Could you check a few things on this model? Use its own coordinates, in mm. A direction names the side the tool comes from. Give positions to 0.01 mm unless a question says otherwise; leave off trailing zeros. Loops run counter-clockwise (first coordinate to the right, second up) from the corner with the lowest first, then second, coordinate; pieces in that order, holes last. Notation, with made-up numbers: (52.5, 25.25) - (77.5, 25.25) arc R20 cw to (77.5, 58.25) - close; hole circle Ø5 at (58, 88). An arc over 180 degrees is marked (long way). Write each question's results on one line, items separated by ' | '. Start each with the question number.
(1) Suppose I cut it at A-A (x = -39). Please give me the cut outline in (y, z).
(2) For pin 1 (1.8 mm diameter, centred on y = 1.5, z = 12, fed in from -X); pin 2 (10 mm diameter, centred on x = -12.5, z = 27.5, fed in from -Y); pin 3 (3 mm diameter, centred on y = 4, z = 47, fed in from +X); pin 4 (1.8 mm diameter, centred on x = -40.5, y = 4.5, fed in from +Z), each with a flat end and sliding along its axis, tell me the tip position at first contact or that it passes through.
(3) Suppose I cut it at C-C (x = 10.5). Please give me the cut outline in (y, z).
(4) I need wall thicknesses on line 1 (Z direction, x = -1.5, y = 3.7); line 2 (Z direction, x = -11.7, y = 4.4); line 3 (Z direction, x = 10.5, y = 1.55). Which ranges of each line are inside material? Lowest first, please.
(5) Suppose I cut it at B-B (x = -11.7). Please give me the cut outline in (y, z).
(6) On a 3-axis mill with a long thin cutter (end or side, diameter ignored), from which of +Z, -Z, +X, -X, +Y, -Y can I reach the whole of each face in a straight line? I mean faces 4 (the face through (-33, 3, 27)), 5 (the face through (-38, 3, 13)), 6 (the face through (0, 3, 54)), 7 (the face through (0, 3, 3)), 8 (the face through (7, 3, 20)). Say none if no direction works.
(7) Suppose I cut it at D-D (z = 30.5). Please give me the cut outline in (x, y), and give its area (3 significant figures).
(8) If we mould it in two halves opening along X, with no side actions, what happens to faces 1 (the face through (19, 3, 31)), 2 (the face through (-41, 3, 21)), 3 (the face through (10.37, 3.042, 37.545))? For each: released by +X, released by -X, zero draft, split by the parting line, or undercut.
Autodesk Inventor part; units mm, degrees
ref_plane "YZ Plane" through (0, 0, 0) normal (1, 0, 0) x (0, 1, 0)
ref_plane "XZ Plane" through (0, 0, 0) normal (0, 1, 0) x (-1, 0, 0)
ref_plane "XY Plane" through (0, 0, 0) normal (0, 0, 1) x (1, 0, 0)
sketch "Sketch1" plane through (0, 0, 0) normal (0, 1, 0) x (-1, 0, 0)
  line L0 (0, 0) -> (38, 0)
  line L1 (44, 0) -> (44, 6)
  line L2 (44, 27) -> (38, 27)
  line L3 (0, 27) -> (0, 6) construction
  line L4 (44, 27) -> (38, 27)
  line L5 (38, 27) -> (38, 21) construction
  line L6 (38, 21) -> (44, 21)
  line L7 (44, 21) -> (44, 27)
  line L8 (44, 0) -> (38, 0)
  line L9 (38, 0) -> (38, 6) construction
  line L10 (38, 6) -> (44, 6)
  line L11 (44, 6) -> (44, 0)
  line L12 (44, 21) -> (44, 27)
  line L13 (38, 27) -> (6, 27)
  line L14 (38, 0) -> (44, 0)
  line L15 (44, 6) -> (44, 21) construction
  line L16 (38, 6) -> (38, 21)
  line L17 (0, 0) -> (6, 0)
  line L18 (6, 0) -> (6, 6) construction
  line L19 (6, 6) -> (0, 6)
  line L20 (0, 6) -> (0, 0)
  line L21 (6, 6) -> (6, 27)
  line L22 (6, 27) -> (0, 27) construction
  line L23 (0, 6) -> (0, 0)
  line L24 (6, 27) -> (21, 27)
  line L25 (21, 27) -> (21, 57)
  line L26 (21, 57) -> (6, 57)
  line L27 (6, 57) -> (0, 57)
  line L28 (0, 57) -> (0, 51)
  line L29 (0, 51) -> (6, 51)
  line L30 (6, 51) -> (6, 57) construction
  line L31 (6, 51) -> (6, 27)
  line L32 (6, 42) -> (-19, 42)
  line L33 (-19, 42) -> (-19, 20)
  line L34 (-19, 20) -> (6, 20)
  line L35 (6, 20) -> (6, 42)
  dimension "d0" = 44
  dimension "d1" = 27
  dimension "d2" = 6
  dimension "d3" = 6
  dimension "d4" = 6
  dimension "d5" = 6
  dimension "d6" = 6
  dimension "d7" = 6
  dimension "d10" = 15
  dimension "d11" = 30
  dimension "d12" = 6
  dimension "d13" = 6
  dimension "d34" = 25
  dimension "d35" = 22
  dimension "d36" = 9
extrude "Extrusion1" add sketch "Sketch1" along normal blind 6
sketch "Sketch2" plane through (0, 6, 0) normal (0, 1, 0) x (1, 0, 0)
  circle A0 centre (10.5, -38.536) radius 1
  circle A1 centre (10.5, -35.536) radius 1
  circle A2 centre (10.5, -32.536) radius 1
  circle A3 centre (-11.7, -28.236) radius 1
  circle A4 centre (-11.7, -25.236) radius 1
  circle A5 centre (-11.7, -22.236) radius 1
  line L0 (0, -51) -> (-6, -51)
  line L1 (19, -42) -> (19, -20)
  dimension "d22" = 2
  dimension "d24" = 2
  dimension "d25" = 3
  dimension "d26" = 2
  dimension "d27" = 3
  dimension "d28" = 2
  dimension "d29" = 2
  dimension "d30" = 3
  dimension "d31" = 2
  dimension "d32" = 3
  dimension "d37" = 10.3
  dimension "d39" = 22.2
  dimension "d51" = 12.464
  dimension "d57" = 8.5
extrude "Extrusion2" cut sketch "Sketch2" against normal through all
properties part number "thumper-bumper-sidewall3-v3"
Output values:
1) outline: (0, 0) - (6, 0) - (6, 6) - (0, 6) - close; (0, 21) - (6, 21) - (6, 27) - (0, 27) - close
2) pin 1: x = -38 | pin 2: y = 0 | pin 3: x = -6 | pin 4: z = 27
3) outline: (0, 20) - (6, 20) - (6, 31.54) - (0, 31.54) - close; (0, 33.54) - (6, 33.54) - (6, 34.54) - (0, 34.54) - close; (0, 36.54) - (6, 36.54) - (6, 37.54) - (0, 37.54) - close; (0, 39.54) - (6, 39.54) - (6, 42) - (0, 42) - close
4) line 1: 0 to 6, 20 to 42, 51 to 57 | line 2: 0 to 21.24, 23.24 to 24.24, 26.24 to 27.24, 29.24 to 57 | line 3: 20 to 31.54, 33.54 to 34.54, 36.54 to 37.54, 39.54 to 42
5) outline: (0, 0) - (6, 0) - (6, 21.24) - (0, 21.24) - close; (0, 23.24) - (6, 23.24) - (6, 24.24) - (0, 24.24) - close; (0, 26.24) - (6, 26.24) - (6, 27.24) - (0, 27.24) - close; (0, 29.24) - (6, 29.24) - (6, 57) - (0, 57) - close
6) face 4: +Z, -X, +Y, -Y | face 5: -X, +Y, -Y | face 6: +Z, +X, +Y, -Y | face 7: -Z, +X, +Y, -Y | face 8: +X, +Y, -Y
7) outline: (-21, 0) - (19, 0) - (19, 6) - (-21, 6) - close | area: 240 mm2
8) face 1: released by +X | face 2: zero draft | face 3: undercut
